Autodesk Inventor part; units mm, degrees
ref_plane "YZ Plane" through (0, 0, 0) normal (1, 0, 0) x (0, 1, 0)
ref_plane "XZ Plane" through (0, 0, 0) normal (0, 1, 0) x (-1, 0, 0)
ref_plane "XY Plane" through (0, 0, 0) normal (0, 0, 1) x (1, 0, 0)
sketch "Sketch1" plane through (0, 0, 0) normal (0, 0, 1) x (1, 0, 0)
  circle A0 centre (0, 0) radius 7.5
  dimension "Diameter" = 15
extrude "Extrusion1" add sketch "Sketch1" along normal blind 37.55
sketch "Sketch2" plane through (0, 0, 37.55) normal (0, 0, 1) x (1, 0, 0)
  circle A0 centre (0, 0) radius 5
  circle A1 centre (0, 0) radius 7.5
  dimension "d3" = 10
extrude "Extrusion2" cut sketch "Sketch2" against normal blind 25
chamfer "Chamfer1" distance 0.1 angle 45 1 edges at (-5, 0, 37.55)
thread "Thread1"
sketch "Sketch3" plane through (0, 0, 0) normal (0, 0, -1) x (-1, 0, 0)
  circle A0 centre (0, 0) radius 5
  circle A1 centre (0, 0) radius 7.5
  dimension "d11" = 10
extrude "Extrusion3" cut sketch "Sketch3" against normal blind 5.5
sketch "Sketch4" plane through (0, 0, 0) normal (0, 0, -1) x (-1, 0, 0)
  point P0 (0, 0)
  point P1 (0, 0)
hole "Hole1" at (0, 0, 0) direction (0, 0, 1) diameter 4.917 depth 12 tip angle 118
chamfer "Chamfer2" distance 0.2 angle 45 3 edges at (5, 0, 0) (-7.5, 0, 5.5) (-7.5, 0, 12.55)
properties part number "Pully Shaft" material "Steel, Alloy"
Geometry check sheet. Reference: the model listing, model coordinates, mm. A direction names the side the tool comes from. Give positions to 0.01 mm unless a question says otherwise; leave off trailing zeros. Loops run counter-clockwise (first coordinate to the right, second up) from the corner with the lowest first, then second, coordinate; pieces in that order, holes last. Notation, with made-up numbers: (-3, 19) -> (4, 19) arc R33 cw to (4, 55) -> close; hole circle Ø3 at (8.25, 61). An arc over 180 degrees is marked (long way). Answer in a Markdown table with one row per item. Add a question column.
1) Set-up check for faces 1 (the face through (0, 0, 37.55)), 2 (the face through (1.08, -4.88, 2.81)), 3 (the face through (-1.08, -4.88, 25.17)): record each of +Z, -Z, +X, -X, +Y, -Y from which the full face is reachable in a straight line by a thin tool's end or side.
2) Cross-section at A-A on z = 10.5. Record the boundary of the cut face in (x, y).
3) Gauge pin test, flat ends, axial feed: P1, Ø4, axis at x = 3, y = 5.5, coming from the +Z side; P2, Ø2, axis at y = 0, z = 14.5, coming from the -X side; P3, Ø1.5, axis at x = 1.5, z = 24, coming from the -Y side. Record the tip position at first contact, or that the pin passes through.
4) Material ranges on probe 1 along Y at (x, z) = (0, 4.5); probe 2 along Y at (x, z) = (0, 9); probe 3 along Z at (x, y) = (1.75, -4.75), recorded low to high. Write a range as from..to.
5) Draft check along Y on faces 4 (the face through (-7.493, -0.33, 8.978)), 5 (the face through (-2, -5, 5.5)), 6 (the face through (-0.164, 0.394, 13.221)). Enter one of: pulls with the +Y half, pulls with the -Y half, needs draft (parallel to the pull), parting line crosses it, or undercut.
6) Cross-section at C-C on z = 4. Record the boundary of the cut face in (x, y), and give its area (3 significant figures).
7) Cross-section at B-B on z = 34. Record the boundary of the cut face in (x, y).
Outcome:
| question | item | result |
|---|---|---|
| 1 | face 1 | +Z, +X, -X, +Y, -Y |
| 1 | face 2 | -Z |
| 1 | face 3 | +Z |
| 2 | outline | circle Ø15 at (0, 0); hole circle Ø4.92 at (0, 0) |
| 3 | P1 | stops at z = 37.55 |
| 3 | P2 | stops at x = -5 |
| 3 | P3 | stops at y = -4.94 |
| 4 | probe 1 | y = -5..-2.46, 2.46..5 |
| 4 | probe 2 | y = -7.5..-2.46, 2.46..7.5 |
| 4 | probe 3 | z = 5.5..12.55 |
| 5 | face 4 | parting line crosses it |
| 5 | face 5 | needs draft |
| 5 | face 6 | undercut |
| 6 | outline | circle Ø10 at (0, 0); hole circle Ø4.92 at (0, 0) |
| 6 | area | 59.6 mm^2 |
| 7 | outline | circle Ø10 at (0, 0) |
